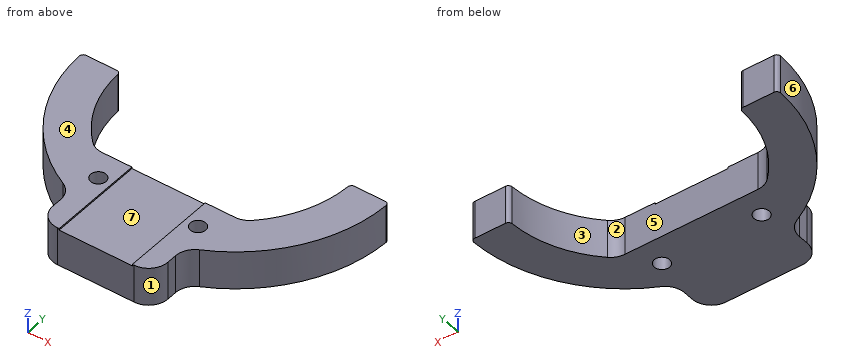
from build123d import *

# Parameters (mm, degrees)
F1_DEPTH = 10
F2_W     = 19.1
F2_H     = 25
F3_DEPTH = 0.4
F4_R     = 2
F5_DEPTH = 10.001
F6_R     = 5
F7_R     = 1


with BuildPart() as f1:
    # F0 (on Top) → F1 (new body)
    with BuildSketch(Plane.XY):
        with BuildLine():
            Line((-30, 0), (-40, 0))
            ThreePointArc((-40, 0), (-33.166248, -22.36068), (-15, -37.080992))
            Line((-15, -37.080992), (-15, -48))
            Line((-15, -48), (15, -48))
            Line((15, -48), (15, -37.080992))
            ThreePointArc((15, -37.080992), (33.166248, -22.36068), (40, 0))
            Line((40, 0), (30, 0))
            ThreePointArc((30, 0), (27.18309, -12.691714), (19.26136, -23))
            Line((19.26136, -23), (-19.26136, -23))
            ThreePointArc((-19.26136, -23), (-27.18309, -12.691714), (-30, 0))
        make_face()
    extrude(amount=F1_DEPTH)

    # F2 (on face) → F3 (cut)
    with BuildSketch(Plane.XY.offset(10)):
        with Locations((0, -35.5)):
            Rectangle(F2_W, F2_H)
    extrude(amount=-F3_DEPTH, mode=Mode.SUBTRACT)

    # F4 (on face) → F5 (cut, through all)
    with BuildSketch(Plane.XY.offset(10)):
        with Locations((-13, -30)):
            Circle(F4_R)
        with Locations((13, -30)):
            Circle(F4_R)
    extrude(amount=-F5_DEPTH, mode=Mode.SUBTRACT)

    # F6
    f6_edges = [f1.edges().sort_by_distance(p)[0] for p in [
        (-19.26136, -23, 5),
        (19.26136, -23, 5),
        (15, -37.080992, 5),
        (-15, -37.080992, 5),
        (-15, -48, 5),
        (15, -48, 5),
    ]]
    fillet(f6_edges, radius=F6_R)

    # F7
    f7_edges = [f1.edges().sort_by_distance(p)[0] for p in [
        (-40, 0, 5),
        (-30, 0, 5),
        (30, 0, 5),
        (40, 0, 5),
    ]]
    fillet(f7_edges, radius=F7_R)


solid = f1.part
Design review of the part built by this model. Coordinates are the model's own, in mm. Face numbers are marked on the shaded views. A direction names the side the tool comes from. Give positions to 0.01 mm unless a question says otherwise; leave off trailing zeros. Loops run counter-clockwise (first coordinate to the right, second up) from the corner with the lowest first, then second, coordinate; pieces in that order, holes last. Notation, with made-up numbers: (60.5, 8) - (115.5, 8) arc R12 cw to (115.5, 15) - close; hole circle Ø3 at (-23.5, 34). An arc over 180 degrees is marked (long way). Use CSV: the item, a comma, the result in double quotes. Start each with the question number.
1. Add section B-B (z = 8.75). State the section outline as (x, y) points, plus the area to 3 significant figures.
2. Machinability: for the marked faces 5, 6 and 7, which of the approach directions +Z, -Z, +X, -X, +Y, -Y give a long, thin tool a straight path to every point of the face, cutting with its end or side? Answer none if there is none.
3. Add section C-C (y = -12). State the section outline as (x, z) points, plus the area to 3 significant figures.
4. Add section D-D (y = -30). State the section outline as (x, z) points.
5. Add section A-A (x = -13). State the section outline as (y, z) points, plus the area to 3 significant figures.
6. Draft analysis for pull direction X (two halves, no side actions). For the marked faces 1, 2, 3 and 4, state which applies: released by +X, released by -X, zero draft, split by the parting line, or undercut.
7. Insertion check: P1, Ø3, axis at x = -20.5, z = 1.5, coming from the -Y side; P2, Ø5, axis at y = -35.5, z = 2.5, coming from the +X side; P3, Ø1.5, axis at y = -30, z = 6, coming from the -X side; P4, Ø15.5, axis at x = 2.5, y = -36.5, coming from the +Z side. Each pin has a flat end and moves straight along its axis. Give the tip position at first contact, or say it passes through.
8. Wall thickness on L1, parallel to X at y = -31, z = 2.5; L2, parallel to Z at x = 9, y = -30; L3, parallel to Y at x = -8, z = 4.5: over which ranges is each line inside the solid? List them lowest first.
Results found:
1,outline,"(-39.99, -1.03) arc R40 ccw to (-17.78, -35.83) arc R5 cw to (-15, -40.31) - (-15, -43) arc R5 ccw to (-10, -48) - (10, -48) arc R5 ccw to (15, -43) - (15, -40.31) arc R5 cw to (17.78, -35.83) arc R40 ccw to (39.99, -1.03) arc R1 ccw to (38.99, 0) - (30.98, 0) arc R1 ccw to (29.98, -0.97) arc R30 cw to (20.82, -21.6) arc R5 cw to (17.35, -23) - (-17.35, -23) arc R5 cw to (-20.82, -21.6) arc R30 cw to (-29.98, -0.97) arc R1 ccw to (-30.98, 0) - (-38.99, 0) arc R1 ccw to start; hole circle Ø4 at (-13, -30); hole circle Ø4 at (13, -30)"
1,area,"1,520 mm²"
2,face 5,"+Z, -Z, +Y"
2,face 6,"+Z, -Z, -X, -Y"
2,face 7,"+Z, +Y, -Y"
3,outline,"(-38.16, 0) - (-27.5, 0) - (-27.5, 10) - (-38.16, 10) - close; (27.5, 0) - (38.16, 0) - (38.16, 10) - (27.5, 10) - close"
3,area,"213 mm²"
4,outline,"(-26.46, 0) - (-15, 0) - (-15, 10) - (-26.46, 10) - close; (-11, 0) - (11, 0) - (11, 10) - (9.55, 10) - (9.55, 9.6) - (-9.55, 9.6) - (-9.55, 10) - (-11, 10) - close; (15, 0) - (26.46, 0) - (26.46, 10) - (15, 10) - close"
5,outline,"(-47, 0) - (-32, 0) - (-32, 10) - (-47, 10) - close; (-28, 0) - (-23, 0) - (-23, 10) - (-28, 10) - close"
5,area,"200 mm²"
6,face 1,"released by +X"
6,face 2,"undercut"
6,face 3,"undercut"
6,face 4,"zero draft"
7,P1,"stops at y = -35.2"
7,P2,"stops at x = 22.61"
7,P3,"stops at x = -27.28"
7,P4,"stops at z = 10"
8,L1,"x = -25.28 to -14.73, -11.27 to 11.27, 14.73 to 25.28"
8,L2,"z = 0 to 9.6"
8,L3,"y = -48 to -23"
